Read the model definition and answer for the solid it produces. Units are mm, in the model's axes. A direction names the side the tool comes from. Coordinates: 2 decimals unless noted, no trailing zeros. Write each loop counter-clockwise with the first axis right and the second up, starting at its lowest first coordinate (ties: lowest second). Pieces come first, ordered by that corner, then holes. Notation, with made-up numbers: (21, -3) - (36, -3) arc R34 cw to (36, 33) - close; hole circle Ø5 at (-22.75, 21.25). An arc over 180 degrees is marked (long way). Return JSON: item names as keys, results as strings.
```python
from build123d import *

# Parameters (mm, degrees)
DOME1_FACE_RADIUS  = 3.302
DOME1_HEIGHT       = 2.54
CUT_EXTRUDE1_DEPTH = 21.698272826
SEED_CUT_COUNT     = 8


# Read off the part's stored shape, not the designer's step: Cut-Revolve-Thin1
with BuildPart() as part:
    # Sketch1 → Revolve1 (revolve)
    with BuildSketch(Plane(origin=(0, 0, 0), x_dir=(0, 0, -1), z_dir=(1, 0, 0)), mode=Mode.PRIVATE) as revolve1_sk:
        Polygon((0, 0), (0, 7.493), (2.54, 7.493), (2.54, 5.08), (15.24, 5.08), (15.24, 0), align=None)
    revolve(revolve1_sk.sketch.rotate(Axis((0, 0, 12.712464269), (0, 0, -1)), 90), axis=Axis((0, 0, 12.712464269), (0, 0, -1)))

    # Sketch2 → Revolve2 (revolve)
    with BuildSketch(Plane(origin=(0, 0, 0), x_dir=(0, 0, -1), z_dir=(1, 0, 0))):
        with BuildLine():
            Line((0, 0), (-7.597075699, 0))
            add(Edge.make_bspline(
                [(0, 5.913009527), (-6.698434988, 5.682543743), (-7.597075699, 0)],
                knots=[0, 0, 0, 1, 1, 1], degree=2))
            Line((0, 5.913009527), (0, 0))
        make_face()
    revolve(axis=Axis((0, 0, 12.712464269), (0, 0, 1)))

    # Cut-Revolve-Thin1 outline → Cut-Revolve-Thin1 (revolve, cut)
    with BuildSketch(Plane.XZ):
        Polygon((5.08, -8.89), (3.302, -13.462), (3.302, -15.24), (5.08, -15.24), align=None)
    revolve(axis=Axis((0, 0, 0), (0, 0, 1)), mode=Mode.SUBTRACT)

    # Dome1: a dome of height H over a round flat face of radius A is a cap of a sphere of radius (A * A + H * H) / (2 * H)
    dome1_r = (DOME1_FACE_RADIUS * DOME1_FACE_RADIUS + DOME1_HEIGHT * DOME1_HEIGHT) / (2 * DOME1_HEIGHT)
    dome1_base = Plane((0, 0, -15.24), z_dir=(0, 0, -1))
    with Locations(dome1_base.offset(DOME1_HEIGHT - dome1_r)):
        dome1_ball = Sphere(dome1_r, mode=Mode.PRIVATE)
    add(split(dome1_ball, bisect_by=dome1_base, keep=Keep.TOP, mode=Mode.PRIVATE))

    # Sketch4 → Cut-Extrude1 (cut, through all)
    with BuildSketch(Plane.XY):
        with BuildLine():
            Line((0, 6.703004763), (0.752149198, 7.455153961))
            ThreePointArc((0.752149198, 7.455153961), (0, 7.493), (-0.752149198, 7.455153961))
            Line((-0.752149198, 7.455153961), (0, 6.703004763))
        make_face()
    cut_extrude1 = extrude(amount=-CUT_EXTRUDE1_DEPTH, mode=Mode.SUBTRACT)

    # Seed Cut: Cut-Extrude1 ×8 about axis
    seed_cut_axis = Axis((0, 0, 0), (0, 0, 1))
    for i in range(1, SEED_CUT_COUNT):
        add(cut_extrude1.rotate(seed_cut_axis, i * 360 / SEED_CUT_COUNT), mode=Mode.SUBTRACT)


solid = part.part
```
(1) Flat-ended cylindrical pins translate along their axes: P1, Ø0.9, axis at y = -5, z = -0.5, coming from the +X side; P2, Ø0.5, axis at y = 5.5, z = -0.5, coming from the -X side; P3, Ø1.5, axis at x = -1.5, y = -0.5, coming from the -Z side. Find the tip coordinate at first contact, or state that the pin passes through.
Answer:
{"P1": "x = 5.95", "P2": "x = -4.74", "P3": "z = -17.68"}
(2) A cutting plane is placed at A-A (z = -11.75). Determine the outline of the cut face in (x, y).
Answer:
{"outline": "circle Ø7.94 at (0, 0)"}
(3) Straight lines are drawn through the part: line 1 (Z direction, x = 5.5, y = -3); line 2 (Z direction, x = 2.5, y = 2.75); line 3 (Y direction, x = -0.5, z = -7.5). For each, find the intervals that lie inside material, in ascending order. Write a range as from..to.
Answer:
{"line 1": "-2.54..0", "line 2": "-12.4..5.91", "line 3": "-5.06..5.06"}
(4) Which of the six approach directions +Z, -Z, +X, -X, +Y, -Y give full straight-line access (tool end or side, diameter ignored) to faces 1 (the face through (-4.74, 5, -1)), 2 (the face through (4.74, -5, -1)), 3 (the face through (5, 4.74, -1)), 4 (the face through (-0.661, -5.037, -5.759))?
Answer:
{"face 1": "+Z, -Z, -X, +Y", "face 2": "+Z, -Z, +X, -Y", "face 3": "+Z, -Z, +X, +Y", "face 4": "-Z"}
